Answer from the drawing. Dimensions are ordinates in mm from the lowest x, y and z of the part. A direction names the side the tool comes from. Round coordinates to 2 decimals unless told otherwise and drop trailing zeros. Loops run counter-clockwise (first coordinate to the right, second up) from the corner with the lowest first, then second, coordinate; pieces in that order, holes last. Notation, with made-up numbers: (63, -34.75) - (114, -34.75) arc R27 cw to (114, -15.75) - close; hole circle Ø1 at (-34.5, 50.25). An arc over 180 degrees is marked (long way). Answer as CSV lines item,"result". Start each with the question number.
Q1. Each of these flat-tipped pins is pushed along its axis until it touches: pin 1 Ø1.5 at (x, y) = (6, 6) entering from -Z; pin 2 Ø3 at (x, y) = (12.5, 10.5) entering from -Z; pin 3 Ø3 at (x, y) = (14, 17.5) entering from -Z; pin 4 Ø25 at (x, y) = (35.5, 33) entering from +Z. Where does it stop, or does it pass through?
Q2. For the marked faces 1 and 2, determine the directions among +Z, -Z, +X, -X, +Y, -Y from which every point of the face is accessible in a straight line to the end or side of a thin tool.
Q3. Straight lines are drawn through the part: L1, parallel to Z at x = 29.5, y = 32.5; L2, parallel to Z at x = 38.5, y = 29; L3, parallel to X at y = 34, z = 5.75. For each, find the intervals that lie inside material, in ascending order. Write a range as [from, to].
Q4. Section B-B on z = 2 is taken. Write down the section's boundary in (x, y), then the cut area to 3 significant figures.
Q5. Section A-A on x = 25 is taken. Write down the section's boundary in (y, z).
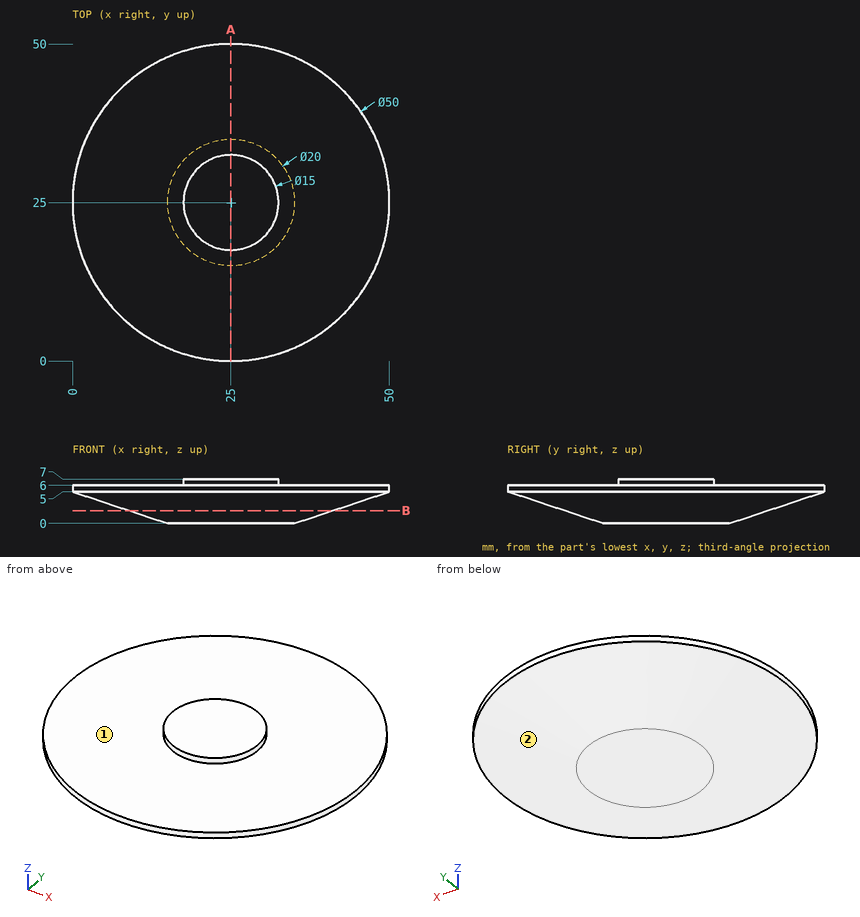
Findings:
1,pin 1,"passes through"
1,pin 2,"stops at z = 2.55"
1,pin 3,"stops at z = 0.6"
1,pin 4,"stops at z = 7"
2,face 1,"+Z"
2,face 2,"-Z"
3,L1,"z = [0, 6]"
3,L2,"z = [1.36, 6]"
3,L3,"x = [1.68, 48.32]"
4,outline,"circle Ø32 at (25, 25)"
4,area,"804 mm^2"
5,outline,"(0, 5) - (15, 0) - (35, 0) - (50, 5) - (50, 6) - (32.5, 6) - (32.5, 7) - (17.5, 7) - (17.5, 6) - (0, 6) - close"
